Verification items for the finished model (mm, model axes). A direction names the side the tool comes from. Round coordinates to 2 decimals unless told otherwise and drop trailing zeros. Write each loop counter-clockwise with the first axis right and the second up, starting at its lowest first coordinate (ties: lowest second). Pieces come first, ordered by that corner, then holes. Notation, with made-up numbers: (72.25, 79) -> (99.25, 79) arc R21 ccw to (99.25, 117) -> close; hole circle Ø4 at (67.25, -8.5). An arc over 180 degrees is marked (long way). Answer as a JSON object with one key per item and string values. Group by question number.
(1) Scan lines: L1, parallel to Y at x = -25, z = 2.85; L2, parallel to X at y = -52.5, z = 3.5; L3, parallel to Y at x = -31, z = 4.85. Record each from-to range of solid material in increasing order. Write a range as from..to.
(2) Sectioned sample at A-A on x = -25. Record the cut outline in (y, z).
(3) Sectioned sample at D-D on x = 9.5. Record the cut outline in (y, z), and give its area (3 significant figures).
(4) Draft check along X on faces 6 (the face through (-17, -55, 2)), 7 (the face through (-24.9, -58.5, 2.5)), 8 (the face through (-27, 54, 3)), 9 (the face through (45, -1, 2)). Enter one of: released by +X, released by -X, zero draft, split by the parting line, or undercut.
(5) Sectioned sample at C-C on y = -52.5. Record the cut outline in (x, z), and give its area (3 significant figures).
(6) Sectioned sample at B-B on z = 3.7. Record the cut outline in (x, y).
(7) Set-up check for faces 1 (the face through (-1, 1, 0)), 2 (the face through (15, 50, 2)), 3 (the face through (-15, -52, 3)), 4 (the face through (-35, 52, 3)), 5 (the face through (-35, -52, 3)): record each of +Z, -Z, +X, -X, +Y, -Y from which the full face is reachable in a straight line by a thin tool's end or side.
(8) Gauge pin test, flat ends, axial feed: pin 1 Ø2.5 at (y, z) = (51.5, 2.5) entering from -X; pin 2 Ø1.5 at (x, z) = (6, 3.5) entering from -Y; pin 3 Ø1.5 at (x, z) = (19, 2) entering from +Y; pin 4 Ø8 at (x, y) = (-25, -52.5) entering from -Z. Record the tip position at first contact, or that the pin passes through.
```python
from build123d import *

# Parameters (mm, degrees)
SKETCH1_W           = 90
SKETCH1_H           = 100
BOSS_EXTRUDE1_DEPTH = 5
SKETCH2_W           = 20
SKETCH2_H           = 5
BOSS_EXTRUDE2_DEPTH = 5
SKETCH3_R           = 6
BOSS_EXTRUDE3_DEPTH = 5
SKETCH4_R           = 2.5
CUT_EXTRUDE1_DEPTH  = 5


with BuildPart() as part:
    # Sketch1 → Boss-Extrude1 (new body)
    with BuildSketch(Plane.XY):
        Rectangle(SKETCH1_W, SKETCH1_H)
    extrude(amount=BOSS_EXTRUDE1_DEPTH)

    # Sketch2 → Boss-Extrude2 (add)
    with BuildSketch(Plane(origin=(0, 50, 0), x_dir=(1, 0, 0), z_dir=(0, 1, 0))):
        with Locations((-25, -2.5)):
            Rectangle(SKETCH2_W, SKETCH2_H)
    boss_extrude2 = extrude(amount=BOSS_EXTRUDE2_DEPTH)

    # Mirror1: Boss-Extrude2 across plane
    add(boss_extrude2.mirror(Plane.ZX))

    # Sketch3 → Boss-Extrude3 (add)
    with BuildSketch(Plane.XY.offset(5)):
        with Locations((-25, 52.5)):
            Circle(SKETCH3_R)
    boss_extrude3 = extrude(amount=-BOSS_EXTRUDE3_DEPTH)

    # Sketch4 → Cut-Extrude1 (cut)
    with BuildSketch(Plane.XY.offset(5)):
        with Locations((-25, 52.5)):
            Circle(SKETCH4_R)
    cut_extrude1 = extrude(amount=-CUT_EXTRUDE1_DEPTH, mode=Mode.SUBTRACT)

    # Mirror2: Boss-Extrude3, Cut-Extrude1 across plane
    add(boss_extrude3.mirror(Plane.ZX))
    add(cut_extrude1.mirror(Plane.ZX), mode=Mode.SUBTRACT)


solid = part.part
```
Computed values:
{
 "1": {"L1": "-58.5..-55, -50..50, 55..58.5", "L2": "-35..-27.5, -22.5..-15", "L3": "-55..55"},
 "2": {"outline": "(-58.5, 0) -> (-55, 0) -> (-55, 5) -> (-58.5, 5) -> close; (-50, 0) -> (50, 0) -> (50, 5) -> (-50, 5) -> close; (55, 0) -> (58.5, 0) -> (58.5, 5) -> (55, 5) -> close"},
 "3": {"outline": "(-50, 0) -> (50, 0) -> (50, 5) -> (-50, 5) -> close", "area": "500 mm2"},
 "4": {"face 6": "zero draft", "face 7": "split by the parting line", "face 8": "undercut", "face 9": "released by +X"},
 "5": {"outline": "(-35, 0) -> (-27.5, 0) -> (-27.5, 5) -> (-35, 5) -> close; (-22.5, 0) -> (-15, 0) -> (-15, 5) -> (-22.5, 5) -> close", "area": "75.0 mm2"},
 "6": {"outline": "(-45, -50) -> (-35, -50) -> (-35, -55) -> (-30.45, -55) arc R6 ccw to (-19.55, -55) -> (-15, -55) -> (-15, -50) -> (45, -50) -> (45, 50) -> (-15, 50) -> (-15, 55) -> (-19.55, 55) arc R6 ccw to (-30.45, 55) -> (-35, 55) -> (-35, 50) -> (-45, 50) -> close; hole circle Ø5 at (-25, -52.5); hole circle Ø5 at (-25, 52.5)"},
 "7": {"face 1": "-Z, +X, -X, +Y, -Y", "face 2": "+Z, -Z, +X, +Y", "face 3": "+Z, -Z, +X, -Y", "face 4": "+Z, -Z, -X, +Y", "face 5": "+Z, -Z, -X, -Y"},
 "8": {"pin 1": "x = -35", "pin 2": "y = -50", "pin 3": "y = 50", "pin 4": "z = 0"}
}
